Can you work these out from the model? Positions are in its coordinate system, mm. A direction names the side the tool comes from. Give positions to 0.01 mm unless a question says otherwise; leave off trailing zeros. Order: outer loops, then holes, each group sorted by start corner. A loop starts at its lowest first (then second) coordinate and runs counter-clockwise, first axis right, second up. Notation, with made-up numbers: (0, 61) - (57, 61) arc R19 ccw to (57, 84) - close; hole circle Ø6 at (54, 60.25). An arc over 180 degrees is marked (long way). Answer as a JSON object with one key per item and string values.
```python
from build123d import *

# Parameters (mm, degrees)
F1_DEPTH = 32.4
F3_DEPTH = 25
F5_DEPTH = 3.2
F7_DEPTH = 20


# Not quite as in the source:
# - a feature names something its author has since deleted; it is built from what else it names


with BuildPart() as f1:
    # F0 (on Top) → F1 (new body)
    with BuildSketch(Plane.XY):
        with BuildLine():
            Line((85.6374964118, -7.5007802074), (-89.3625035882, -7.5007802074))
            ThreePointArc((-89.3625035882, -7.5007802074), (-92.8980374941, -8.9652463014), (-94.3625035882, -12.5007802074))
            Line((-94.3625035882, -12.5007802074), (-94.3625035882, -36.1007802074))
            ThreePointArc((-94.3625035882, -36.1007802074), (-92.8980374941, -39.6363141133), (-89.3625035882, -41.1007802074))
            add(Edge.make_bspline(
                [(-89.3625035882, -41.1007802074), (-59.4132024584, -34.6381396439), (-0.1322912347, -21.8461476087), (57.2468589299, -34.7273087443), (85.6374964118, -41.1007802074)],
                knots=[0, 0, 0, 0, 0.5052098646, 1, 1, 1, 1], degree=3))
            ThreePointArc((85.6374964118, -41.1007802074), (89.1730303177, -39.6363141133), (90.6374964118, -36.1007802074))
            Line((90.6374964118, -36.1007802074), (90.6374964118, -12.5007802074))
            ThreePointArc((90.6374964118, -12.5007802074), (89.1730303177, -8.9652463014), (85.6374964118, -7.5007802074))
        make_face()
        with BuildLine():
            add(Edge.make_bspline(
                [(-89.3625035882, -41.1007802074), (-59.4132024584, -34.6381396439), (-0.1322912347, -21.8461476087), (57.2468589299, -34.7273087443), (85.6374964118, -41.1007802074)],
                knots=[0, 0, 0, 0, 0.5052098646, 1, 1, 1, 1], degree=3))
            Line((-89.3625035882, -41.1007802074), (85.6374964118, -41.1007802074))
        make_face()
    extrude(amount=F1_DEPTH)

    # F2 (on face) → F3 (cut)
    with BuildSketch(Plane.XY.offset(32.4)):
        with BuildLine():
            add(Edge.make_bspline(
                [(-89.3625035882, -41.1007802074), (-59.456438476, -34.254019451), (-0.1066600814, -25.9658719218), (57.8851377231, -34.2465879534), (86.657191818, -40.9956981105)],
                knots=[0, 0, 0, 0, 0.5038023595, 1, 1, 1, 1], degree=3))
            Line((-89.3625035882, -41.1007802074), (85.6374964118, -41.1007802074))
            ThreePointArc((85.6374964118, -41.1007802074), (86.1500442068, -41.0744403041), (86.657191818, -40.9956981105))
        make_face()
    extrude(amount=-F3_DEPTH, mode=Mode.SUBTRACT)

    # F4 (on face) → F5 (join)
    with BuildSketch(Plane(origin=(0, 0, 0), x_dir=(1, 0, 0), z_dir=(0, 0, -1))):
        with BuildLine():
            Line((-51.5625035882, 18.8695881516), (-54.9125035882, 18.8695881516))
            ThreePointArc((-54.9125035882, 18.8695881516), (-51.5625035882, 15.5195881516), (-48.2125035882, 18.8695881516))
            Line((-48.2125035882, 18.8695881516), (-51.5625035882, 18.8695881516))
        make_face()
        with BuildLine():
            ThreePointArc((-48.2125035882, 18.8695881516), (-51.5625035882, 22.2195881516), (-54.9125035882, 18.8695881516))
            Line((-54.9125035882, 18.8695881516), (-51.5625035882, 18.8695881516))
            Line((-51.5625035882, 18.8695881516), (-48.2125035882, 18.8695881516))
        make_face()
        with BuildLine():
            ThreePointArc((51.1874964118, 18.8695881516), (47.8374964118, 22.2195881516), (44.4874964118, 18.8695881516))
            Line((44.4874964118, 18.8695881516), (47.8374964118, 18.8695881516))
            Line((47.8374964118, 18.8695881516), (51.1874964118, 18.8695881516))
        make_face()
        with BuildLine():
            Line((47.8374964118, 18.8695881516), (44.4874964118, 18.8695881516))
            ThreePointArc((44.4874964118, 18.8695881516), (47.8374964118, 15.5195881516), (51.1874964118, 18.8695881516))
            Line((51.1874964118, 18.8695881516), (47.8374964118, 18.8695881516))
        make_face()
    extrude(amount=F5_DEPTH)

    # F6 (on face) → F7 (cut)
    with BuildSketch(Plane(origin=(0, 0, -3.2), x_dir=(1, 0, 0), z_dir=(0, 0, -1))):
        with BuildLine():
            ThreePointArc((49.7674964118, 18.8695881516), (46.6597964296, 20.3986148851), (47.3447785341, 17.0035417714))
            ThreePointArc((47.3447785341, 17.0035417714), (49.015196394, 17.340561418), (49.7674964118, 18.8695881516))
        make_face()
        with BuildLine():
            ThreePointArc((-52.6547781922, 17.2789104499), (-50.6630550607, 17.1616089388), (-49.6317802739, 18.8695881516))
            ThreePointArc((-49.6317802739, 18.8695881516), (-52.4605054871, 20.5775673643), (-52.6547781922, 17.2789104499))
        make_face()
    extrude(amount=-F7_DEPTH, mode=Mode.SUBTRACT)


solid = f1.part
```
Q1. I need wall thicknesses on L1, parallel to X at y = -17.5, z = 16; L2, parallel to Z at x = 39, y = -29.5; L3, parallel to Z at x = -38.5, y = -33. Which ranges of each line are inside material? Lowest first, please.
Recorded:
{"L1": "x = -94.36 to -52.92, -50.2 to 46.48, 49.2 to 90.64", "L2": "z = 0 to 32.4", "L3": "z = 0 to 7.4"}
Q2. Which directions (+Z, -Z, +X, -X, +Y, -Y) give clear straight access to the entire face, cutting with the end or side of a thin tool? Please do faces 1 (the face through (48, -19, 16.8)), 2 (the face through (-94.363, -24, 16)).
Recorded:
{"face 1": "-Z", "face 2": "+Z, -Z, -X, +Y, -Y"}
Q3. We'd pull the mould along X, two halves only. Please class faces 3 (the face through (90.637, -24, 16)), 4 (the face through (-3, -41.101, 4)), 5 (the face through (44.74, -20.15, -1.58)): released by +X, released by -X, zero draft, split by the parting line, or undercut.
Recorded:
{"face 3": "released by +X", "face 4": "zero draft", "face 5": "undercut"}
Q4. I'm going to push flat-ended pins straight in: pin 1 Ø10 at (x, y) = (26.5, -18.5) entering from -Z; pin 2 Ø4 at (x, z) = (70.5, 22.5) entering from -Y; pin 3 Ø3 at (x, y) = (47.5, -18) entering from -Z; pin 4 Ø2 at (x, z) = (24, 10.5) entering from -Y. Where does each tip first touch, or does it pass through?
Recorded:
{"pin 1": "stops at z = 0", "pin 2": "stops at y = -37.89", "pin 3": "stops at z = -3.2", "pin 4": "stops at y = -31.11"}
Q5. If we section it at B-B, the plane y = -10: Please give me the cut outline in (x, z), then the cut area to 3 significant figures.
Recorded:
{"outline": "(-93.69, 0) - (89.97, 0) - (89.97, 32.4) - (-93.69, 32.4) - close", "area": "5,950 mm^2"}
Q6. If we section it at A-A, the plane y = -25: Please give me the cut outline in (x, z), then the cut area to 3 significant figures.
Recorded:
{"outline": "(-94.36, 0) - (90.64, 0) - (90.64, 32.4) - (-94.36, 32.4) - close", "area": "5,990 mm^2"}
